For this review, take the finished solid that the model builds, in its own axes (mm). Coordinates: 2 decimals unless noted, no trailing zeros. Loops run counter-clockwise (first coordinate to the right, second up) from the corner with the lowest first, then second, coordinate; pieces in that order, holes last. Notation, with made-up numbers: M 24.5,-14.5 L 35.5,-14.5 A22 ccw 35.5,21.5 Z; hole C 28.5,10 d9. An arc over 180 degrees is marked long. Answer as a JSON object with one key per item and string values. Group by question number.
Item 1: Add section C-C (z = 4). State the section outline as (x, y) points, then the cut area to 3 significant figures.
Item 2: Add section A-A (y = 0). State the section outline as (x, z) points.
Item 3: Insertion check: pin 1 (1 mm diameter, centred on y = 0, z = 12.5, fed in from +X). The pin has a flat end and moves straight along its axis. Give the tip position at first contact, or say it passes through.
Item 4: Wall thickness on L1, parallel to Z at x = -0.4, y = -0.5; L2, parallel to Y at x = 0, z = 3.5; L3, parallel to Z at x = 0.7, y = -0.45: over which ranges is each line inside the solid? List them lowest first. Write a range as from..to.
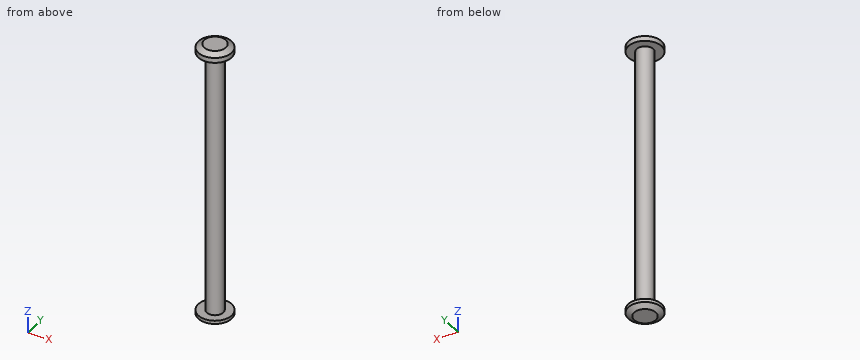
from build123d import *

# Parameters (mm, degrees)
SKETCH1_R           = 0.5
BOSS_EXTRUDE1_DEPTH = 16
SKETCH2_R           = 1
BOSS_EXTRUDE2_DEPTH = 0.4
CHAMFER1_SIZE       = 0.2
CHAMFER1_SIZE2      = 0.346410162
BOSS_EXTRUDE3_START = 0.5
SKETCH3_R           = 1
BOSS_EXTRUDE3_DEPTH = 0.5
CHAMFER2_SIZE       = 0.2
CHAMFER2_SIZE2      = 0.346410162


with BuildPart() as part:
    # Sketch1 → Boss-Extrude1 (new body)
    with BuildSketch(Plane.XY):
        Circle(SKETCH1_R)
    extrude(amount=BOSS_EXTRUDE1_DEPTH)

    # Sketch2 → Boss-Extrude2 (add)
    with BuildSketch(Plane(origin=(0, 0, 0), x_dir=(-1, 0, 0), z_dir=(0, 0, -1))):
        Circle(SKETCH2_R)
    extrude(amount=BOSS_EXTRUDE2_DEPTH)

    # Chamfer1
    chamfer1_edges = [part.edges().sort_by_distance(p)[0] for p in [
        (1, 0, -0.4),
    ]]
    chamfer1_side = [part.faces().sort_by_distance(p)[0] for p in [
        (1, 0, -0.2),
    ]]
    chamfer(chamfer1_edges, length=CHAMFER1_SIZE, length2=CHAMFER1_SIZE2, reference=chamfer1_side[0])

    # Sketch3 → Boss-Extrude3 (add)
    with BuildSketch(Plane.XY.offset(16).offset(BOSS_EXTRUDE3_START)):
        with Locations(Location((0, 0, 0), (0, 0, 180))):
            Circle(SKETCH3_R)
    extrude(amount=-BOSS_EXTRUDE3_DEPTH)

    # Chamfer2
    chamfer2_edges = [part.edges().sort_by_distance(p)[0] for p in [
        (1, 0, 16.5),
    ]]
    chamfer2_side = [part.faces().sort_by_distance(p)[0] for p in [
        (1, 0, 16.25),
    ]]
    chamfer(chamfer2_edges, length=CHAMFER2_SIZE, length2=CHAMFER2_SIZE2, reference=chamfer2_side[0])


solid = part.part
From the geometry:
{
 "1": {"outline": "C 0,0 d1", "area": "0.785 mm²"},
 "2": {"outline": "M -1,-0.2 L -0.65,-0.4 L 0.65,-0.4 L 1,-0.2 L 1,0 L 0.5,0 L 0.5,16 L 1,16 L 1,16.3 L 0.65,16.5 L -0.65,16.5 L -1,16.3 L -1,16 L -0.5,16 L -0.5,0 L -1,0 Z"},
 "3": {"pin 1": "stops at x = 0.5"},
 "4": {"L1": "z = -0.4..0, 16..16.5", "L2": "y = -0.5..0.5", "L3": "z = -0.3..0, 16..16.4"}
}
